Check sheet for the drawn part. Datum: minimum x, y, z corner. Units: mm. Coordinates: 2 decimals unless noted, no trailing zeros. Order: outer loops, then holes, each group sorted by start corner. A loop starts at its lowest first (then second) coordinate and runs counter-clockwise, first axis right, second up. Notation, with made-up numbers: (-33.5, 52) -> (-14.5, 52) arc R18 cw to (-14.5, 85) -> close; hole circle Ø9 at (-33, 44). An arc over 180 degrees is marked (long way). Write item = value, one per line. Start each with the question number.
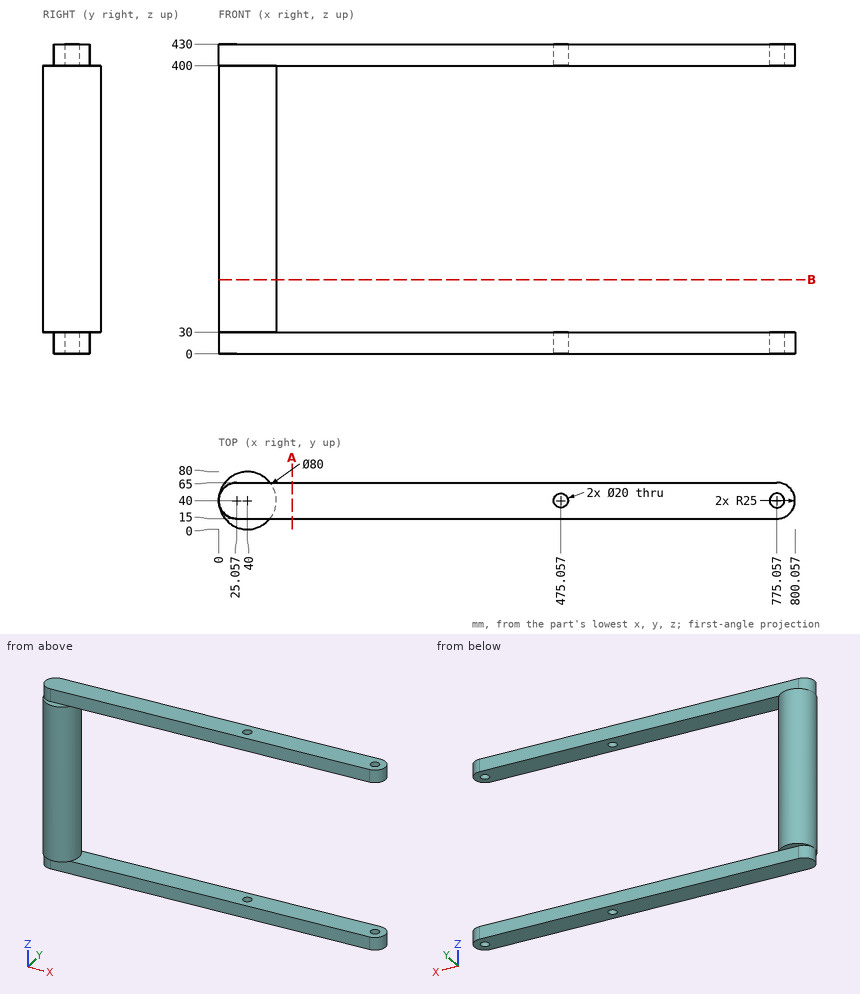
Item 1: Section check A-A (x = 102). Record the boundary of the cut face in (y, z), then the cut area to 3 significant figures.
Item 2: Thickness scan on line 1 (Z direction, x = 284, y = 62.5); line 2 (Y direction, x = 37, z = 104); line 3 (X direction, y = 64, z = 338.5). Record the ranges inside material, lowest first.
Item 3: Gauge pin test, flat ends, axial feed: P1, Ø16, axis at x = 475.06, y = 40, coming from the -Z side; P2, Ø8, axis at y = 46, z = 47.5, coming from the +X side; P3, Ø24, axis at x = 400, z = 414.5, coming from the -Y side; P4, Ø24, axis at x = 288, z = 10, coming from the +Y side. Record the tip position at first contact, or that the pin passes through.
Item 4: Section check B-B (z = 103). Record the boundary of the cut face in (x, y).
Filled sheet:
q1.outline = (15, 0) -> (65, 0) -> (65, 30) -> (15, 30) -> close; (15, 400) -> (65, 400) -> (65, 430) -> (15, 430) -> close
q1.area = 3,000 mm^2
q2.line_1 = 0 to 30, 400 to 430
q2.line_2 = 0.11 to 79.89
q2.line_3 = 8 to 72
q3.P1 = through
q3.P2 = 79.95
q3.P3 = 15
q3.P4 = 65
q4.outline = circle Ø80 at (40, 40)
